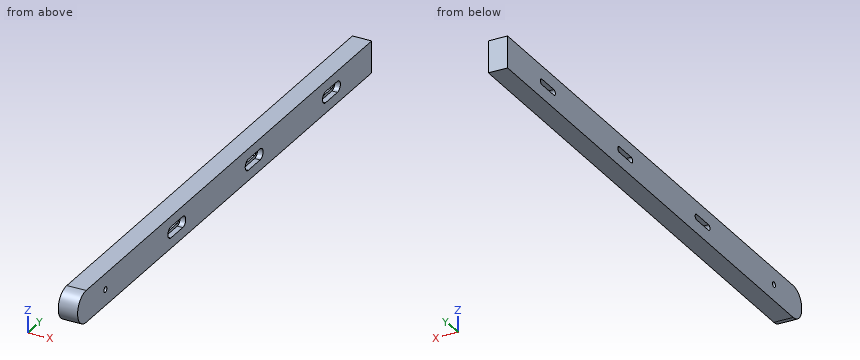
```python
from build123d import *

# Parameters (mm, degrees)
F0_R     = 1.5875
F1_DEPTH = 11.1125
F2_DEPTH = 3.175


with BuildPart() as f1:
    # F0 (on Right) → F1 (new body)
    with BuildSketch(Plane.YZ):
        with BuildLine():
            Line((304.8, 9.128125), (0, 9.128125))
            ThreePointArc((0, 9.128125), (-9.128125, 0), (0, -9.128125))
            Line((0, -9.128125), (0, -9.140291))
            Line((0, -9.140291), (304.8, -9.140291))
            Line((304.8, -9.140291), (304.8, 9.128125))
        make_face()
        with Locations((20.528005, 0)):
            Circle(F0_R, mode=Mode.SUBTRACT)
        with BuildLine():
            Line((103.078005, -3.175), (90.378005, -3.175))
            ThreePointArc((90.378005, -3.175), (87.203005, 0), (90.378005, 3.175))
            Line((90.378005, 3.175), (103.078005, 3.175))
            ThreePointArc((103.078005, 3.175), (106.253005, 0), (103.078005, -3.175))
        make_face(mode=Mode.SUBTRACT)
        with BuildLine():
            Line((185.628005, -3.175), (172.928005, -3.175))
            ThreePointArc((172.928005, -3.175), (169.753005, 0), (172.928005, 3.175))
            Line((172.928005, 3.175), (185.628005, 3.175))
            ThreePointArc((185.628005, 3.175), (188.803005, 0), (185.628005, -3.175))
        make_face(mode=Mode.SUBTRACT)
        with BuildLine():
            Line((268.178005, -3.175), (255.478005, -3.175))
            ThreePointArc((255.478005, -3.175), (252.303005, 0), (255.478005, 3.175))
            Line((255.478005, 3.175), (268.178005, 3.175))
            ThreePointArc((268.178005, 3.175), (271.353005, 0), (268.178005, -3.175))
        make_face(mode=Mode.SUBTRACT)
        with BuildLine():
            ThreePointArc((90.378005, 3.175), (87.203005, 0), (90.378005, -3.175))
            Line((90.378005, -3.175), (103.078005, -3.175))
            ThreePointArc((103.078005, -3.175), (106.253005, 0), (103.078005, 3.175))
            Line((103.078005, 3.175), (90.378005, 3.175))
        make_face()
        with BuildLine():
            Line((103.078005, -1.5875), (90.378005, -1.5875))
            ThreePointArc((90.378005, -1.5875), (88.790505, 0), (90.378005, 1.5875))
            Line((90.378005, 1.5875), (103.078005, 1.5875))
            ThreePointArc((103.078005, 1.5875), (104.665505, 0), (103.078005, -1.5875))
        make_face(mode=Mode.SUBTRACT)
        with BuildLine():
            ThreePointArc((255.478005, 3.175), (252.303005, 0), (255.478005, -3.175))
            Line((255.478005, -3.175), (268.178005, -3.175))
            ThreePointArc((268.178005, -3.175), (271.353005, 0), (268.178005, 3.175))
            Line((268.178005, 3.175), (255.478005, 3.175))
        make_face()
        with BuildLine():
            Line((268.178005, -1.5875), (255.478005, -1.5875))
            ThreePointArc((255.478005, -1.5875), (253.890505, 0), (255.478005, 1.5875))
            Line((255.478005, 1.5875), (268.178005, 1.5875))
            ThreePointArc((268.178005, 1.5875), (269.765505, 0), (268.178005, -1.5875))
        make_face(mode=Mode.SUBTRACT)
        with BuildLine():
            ThreePointArc((172.928005, 3.175), (169.753005, 0), (172.928005, -3.175))
            Line((172.928005, -3.175), (185.628005, -3.175))
            ThreePointArc((185.628005, -3.175), (188.803005, 0), (185.628005, 3.175))
            Line((185.628005, 3.175), (172.928005, 3.175))
        make_face()
        with BuildLine():
            Line((185.628005, -1.5875), (172.928005, -1.5875))
            ThreePointArc((172.928005, -1.5875), (171.340505, 0), (172.928005, 1.5875))
            Line((172.928005, 1.5875), (185.628005, 1.5875))
            ThreePointArc((185.628005, 1.5875), (187.215505, 0), (185.628005, -1.5875))
        make_face(mode=Mode.SUBTRACT)
    extrude(amount=-F1_DEPTH)

    # F0 (on Right) → F2 (cut)
    with BuildSketch(Plane.YZ):
        with BuildLine():
            ThreePointArc((90.378005, 3.175), (87.203005, 0), (90.378005, -3.175))
            Line((90.378005, -3.175), (103.078005, -3.175))
            ThreePointArc((103.078005, -3.175), (106.253005, 0), (103.078005, 3.175))
            Line((103.078005, 3.175), (90.378005, 3.175))
        make_face()
        with BuildLine():
            Line((103.078005, -1.5875), (90.378005, -1.5875))
            ThreePointArc((90.378005, -1.5875), (88.790505, 0), (90.378005, 1.5875))
            Line((90.378005, 1.5875), (103.078005, 1.5875))
            ThreePointArc((103.078005, 1.5875), (104.665505, 0), (103.078005, -1.5875))
        make_face(mode=Mode.SUBTRACT)
        with BuildLine():
            ThreePointArc((172.928005, 3.175), (169.753005, 0), (172.928005, -3.175))
            Line((172.928005, -3.175), (185.628005, -3.175))
            ThreePointArc((185.628005, -3.175), (188.803005, 0), (185.628005, 3.175))
            Line((185.628005, 3.175), (172.928005, 3.175))
        make_face()
        with BuildLine():
            Line((185.628005, -1.5875), (172.928005, -1.5875))
            ThreePointArc((172.928005, -1.5875), (171.340505, 0), (172.928005, 1.5875))
            Line((172.928005, 1.5875), (185.628005, 1.5875))
            ThreePointArc((185.628005, 1.5875), (187.215505, 0), (185.628005, -1.5875))
        make_face(mode=Mode.SUBTRACT)
        with BuildLine():
            ThreePointArc((255.478005, 3.175), (252.303005, 0), (255.478005, -3.175))
            Line((255.478005, -3.175), (268.178005, -3.175))
            ThreePointArc((268.178005, -3.175), (271.353005, 0), (268.178005, 3.175))
            Line((268.178005, 3.175), (255.478005, 3.175))
        make_face()
        with BuildLine():
            Line((268.178005, -1.5875), (255.478005, -1.5875))
            ThreePointArc((255.478005, -1.5875), (253.890505, 0), (255.478005, 1.5875))
            Line((255.478005, 1.5875), (268.178005, 1.5875))
            ThreePointArc((268.178005, 1.5875), (269.765505, 0), (268.178005, -1.5875))
        make_face(mode=Mode.SUBTRACT)
    extrude(amount=-F2_DEPTH, mode=Mode.SUBTRACT)


solid = f1.part
```
Geometry: final body of the model. Coordinates: model frame, mm. Round coordinates to 2 decimals unless told otherwise and drop trailing zeros. Order: outer loops, then holes, each group sorted by start corner. A loop starts at its lowest first (then second) coordinate and runs counter-clockwise, first axis right, second up. Notation, with made-up numbers: (33.25, -1.5) -> (90.25, -1.5) arc R25 cw to (90.25, 28.5) -> close; hole circle Ø6 at (83, 27.5). An arc over 180 degrees is marked (long way). Use one line per item in the form item = value. Start each with the question number.
1. Line query: probe 1 along Z at (x, y) = (-10, 180.5); probe 2 along Y at (x, z) = (-2, -6.5); probe 3 along Y at (x, z) = (-7.5, 5). Output: solid intervals per line, ascending.
2. Pin query (flat end, axial travel): pin 1 Ø1.9 at (y, z) = (99, 1) entering from +X (3 decimals); pin 2 Ø5 at (x, z) = (-4.5, 6) entering from -Y; pin 3 Ø2.5 at (y, z) = (20.53, 0) entering from +X; pin 4 Ø3 at (x, z) = (-6.5, 7) entering from -Y. Return the tip coordinate at first contact, or that it passes through.
3. Cut plane B-B (y = 258.5). Return the cut outline in (x, z) (1 decimal), then the cut area to 3 significant figures.
4. Cut plane A-A (x = -5.25). Count the separate pieces of the cut face and the enclosed holes in it, then the cut area to 3 significant figures.
Solution:
q1.probe_1 = -9.14 to -1.59, 1.59 to 9.13
q1.probe_2 = -6.41 to 304.8
q1.probe_3 = -7.64 to 304.8
q2.pin_1 = -3.175
q2.pin_2 = -8.43
q2.pin_3 = through
q2.pin_4 = -7.29
q3.outline = (-11.1, -9.1) -> (0, -9.1) -> (0, -3.2) -> (-3.2, -3.2) -> (-3.2, -1.6) -> (-11.1, -1.6) -> close; (-11.1, 1.6) -> (-3.2, 1.6) -> (-3.2, 3.2) -> (0, 3.2) -> (0, 9.1) -> (-11.1, 9.1) -> close
q3.area = 158 mm^2
q4.separate_pieces = 1
q4.enclosed_holes = 4
q4.area = 5,550 mm^2
